```python
from build123d import *

# Parameters (mm, degrees)
SKETCH3_R               = 0.65
CUT_EXTRUDE1_DEPTH      = 2
SKETCH4_R               = 0.65
CUT_EXTRUDE2_DEPTH      = 2
SKETCH6_W               = 0.570635025
SKETCH6_H               = 1.87642035
CUT_EXTRUDE4_DEPTH      = 5
CUT_EXTRUDE4_DEPTH_BACK = 5


with BuildPart() as part:
    # Sketch2 → Revolve1 (revolve)
    with BuildSketch(Plane.XY):
        with BuildLine():
            Line((-3.879111396, 0), (-3.879111396, -12))
            add(Edge.make_bspline(
                [(-3.879111396, -12), (-3.879111402, -12.602750297)],
                knots=[0, 0, 1, 1], degree=1))
            add(Edge.make_bspline(
                [(-3.879111402, -12.602750297), (-4.096238593, -15.249180041), (-0.537349984, -14.727809099), (-0.795067133, -17.31657115)],
                knots=[0, 0, 0, 0, 1, 1, 1, 1], degree=3))
            Line((-0.795067133, -17.31657115), (0, -17.31657115))
            Line((0, -17.31657115), (0, 0))
            Line((0, 0), (-3.879111396, 0))
        make_face()
    revolve(axis=Axis((0, 0, 0), (0, -1, 0)))

    # Sketch3 → Cut-Extrude1 (cut)
    with BuildSketch(Plane.XY.offset(3.9)):
        with Locations((0, -1.5)):
            Circle(SKETCH3_R)
    extrude(amount=-CUT_EXTRUDE1_DEPTH, mode=Mode.SUBTRACT)

    # Sketch4 → Cut-Extrude2 (cut)
    with BuildSketch(Plane.XY.offset(-3.9)):
        with Locations((0, -1.5)):
            Circle(SKETCH4_R)
    extrude(amount=CUT_EXTRUDE2_DEPTH, mode=Mode.SUBTRACT)

    # Sketch6 → Cut-Extrude4 (cut, two sides)
    with BuildSketch(Plane(origin=(0, 0, 0), x_dir=(0, 0, -1), z_dir=(1, 0, 0))) as cut_extrude4_sk:
        with Locations((-3.8850644, -1.538047365)):
            Rectangle(SKETCH6_W, SKETCH6_H)
    extrude(amount=CUT_EXTRUDE4_DEPTH, mode=Mode.SUBTRACT)
    extrude(cut_extrude4_sk.sketch, amount=-CUT_EXTRUDE4_DEPTH_BACK, mode=Mode.SUBTRACT)


solid = part.part
```
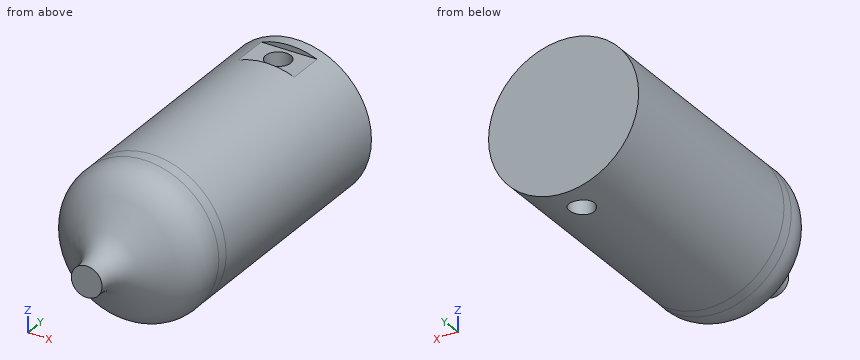
Verification items for the finished model (mm, model axes). Give positions to 0.01 mm unless a question says otherwise; leave off trailing zeros. Order: outer loops, then holes, each group sorted by start corner. A loop starts at its lowest first (then second) coordinate and runs counter-clockwise, first axis right, second up. Notation, with made-up numbers: (-20, 44.25) -> (37, 44.25) arc R18 cw to (37, 66.25) -> close; hole circle Ø11 at (-2, 75). An arc over 180 degrees is marked (long way). Use a Markdown table: item, result.
1) Depth check by flat-ended pin: pin 1 Ø1.4 at (x, y) = (0.5, -1) entering from -Z; pin 2 Ø1.4 at (x, y) = (0, -1) entering from +Z; pin 3 Ø1 at (y, z) = (-7, 1.5) entering from -X. Enter the tip coordinate at first touch or a pass-through.
Results:
| item | result |
|---|---|
| pin 1 | z = -3.88 |
| pin 2 | z = 3.88 |
| pin 3 | x = -3.75 |
2) Material ranges on probe 1 along X at (y, z) = (-11, 0); probe 2 along Y at (x, z) = (0, 3.2); probe 3 along Y at (x, z) = (0, -2.35), recorded low to high.
Results:
| item | result |
|---|---|
| probe 1 | -3.88 to 3.88 |
| probe 2 | -14.35 to -2.15, -0.85 to 0 |
| probe 3 | -14.96 to -2.15, -0.85 to 0 |
3) Section check A-A, the plane y = -4.5. Record the boundary of the cut face in (x, z), then the cut area to 3 significant figures.
Results:
| item | result |
|---|---|
| outline | circle Ø7.76 at (0, 0) |
| area | 47.3 mm² |
